Can you work these out from the model? Positions are in its coordinate system, mm. A direction names the side the tool comes from. Round coordinates to 2 decimals unless told otherwise and drop trailing zeros. Loops run counter-clockwise (first coordinate to the right, second up) from the corner with the lowest first, then second, coordinate; pieces in that order, holes last.
Autodesk Inventor part; units mm, degrees
ref_plane "YZ Plane" through (0, 0, 0) normal (1, 0, 0) x (0, 1, 0)
ref_plane "XZ Plane" through (0, 0, 0) normal (0, 1, 0) x (-1, 0, 0)
ref_plane "XY Plane" through (0, 0, 0) normal (0, 0, 1) x (1, 0, 0)
sketch "스케치1" plane through (0, 0, 0) normal (0, 1, 0) x (-1, 0, 0)
  line L0 (0, 0) -> (-59.6, 0)
  line L1 (-59.6, 0) -> (-59.6, 54.8)
  line L2 (-59.6, 54.8) -> (0, 54.8)
  line L3 (0, 54.8) -> (0, 0)
  dimension "d0" = 59.6
  dimension "d1" = 54.8
extrude "돌출1" add sketch "스케치1" along normal blind 14.7
sketch "스케치3" plane through (0, 14.7, 0) normal (0, 1, 0) x (1, 0, 0)
  line L0 (3.6, -3.85) -> (56, -3.85)
  line L1 (56, -3.85) -> (56, -50.95)
  line L2 (56, -50.95) -> (3.6, -50.95)
  line L3 (3.6, -50.95) -> (3.6, -3.85)
  point P0 (0, 0)
  dimension "d10" = 52.4
  dimension "d11" = 47.1
extrude "돌출2" add sketch "스케치3" along normal blind 7.2
sketch "스케치4" plane through (0, 21.9, 0) normal (0, 1, 0) x (1, 0, 0)
  line L0 (23.4801, -25.2454) -> (33.4417, -25.2454) construction
  line L1 (33.4417, -25.2454) -> (33.4417, -28.4935) construction
  line L2 (33.4417, -28.4935) -> (23.4801, -28.4935) construction
  line L3 (23.4801, -28.4935) -> (23.4801, -25.2454) construction
  line L4 (25.5376, -28.4293) -> (25.1523, -28.4293)
  line L5 (25.1523, -28.4293) -> (25.1523, -28.1773)
  spline S0 degree 2 poles (25.1523, -28.1773) (24.9745, -28.3329) (24.6558, -28.4935) (24.4582, -28.4935) knots 0 0 0 1 2 2 2
  spline S1 degree 2 poles (24.4582, -28.4935) (24.31, -28.4935) (24.0457, -28.3947) (23.9494, -28.2885) knots 0 0 0 1 2 2 2
  spline S2 degree 2 poles (23.9494, -28.2885) (23.8506, -28.1823) (23.7419, -27.8587) (23.7419, -27.6265) knots 0 0 0 1 2 2 2
  line L6 (23.7419, -27.6265) -> (23.7419, -26.142)
  line L7 (23.7419, -26.142) -> (24.1272, -26.142)
  line L8 (24.1272, -26.142) -> (24.1272, -27.4462)
  spline S3 degree 2 poles (24.1272, -27.4462) (24.1272, -27.629) (24.1544, -27.8686) (24.2013, -27.9575) knots 0 0 0 1 2 2 2
  spline S4 degree 2 poles (24.2013, -27.9575) (24.2483, -28.0464) (24.4088, -28.1279) (24.5595, -28.1279) knots 0 0 0 1 2 2 2
  spline S5 degree 2 poles (24.5595, -28.1279) (24.7003, -28.1279) (25.0189, -27.9674) (25.1523, -27.8513) knots 0 0 0 1 2 2 2
  line L9 (25.1523, -27.8513) -> (25.1523, -26.142)
  line L10 (25.1523, -26.142) -> (25.5376, -26.142)
  line L11 (25.5376, -26.142) -> (25.5376, -28.4293)
  spline S6 degree 2 poles (28.0126, -27.2486) (28.0126, -27.8093) (27.4692, -28.4935) (27.0591, -28.4935) knots 0 0 0 1 2 2 2
  spline S7 degree 2 poles (27.0591, -28.4935) (26.8739, -28.4935) (26.6096, -28.4021) (26.4812, -28.3231) knots 0 0 0 1 2 2 2
  line L12 (26.4812, -28.3231) -> (26.4565, -28.4293)
  line L13 (26.4565, -28.4293) -> (26.0958, -28.4293)
  line L14 (26.0958, -28.4293) -> (26.0958, -25.2454)
  line L15 (26.0958, -25.2454) -> (26.4812, -25.2454)
  line L16 (26.4812, -25.2454) -> (26.4812, -26.3816)
  spline S8 degree 2 poles (26.4812, -26.3816) (26.6269, -26.2507) (26.9653, -26.0778) (27.1802, -26.0778) knots 0 0 0 1 2 2 2
  spline S9 degree 2 poles (27.1802, -26.0778) (27.568, -26.0778) (28.0126, -26.6978) (28.0126, -27.2486) knots 0 0 0 1 2 2 2
  spline S10 degree 2 poles (27.6149, -27.2782) (27.6149, -26.8682) (27.3654, -26.4434) (27.0888, -26.4434) knots 0 0 0 1 2 2 2
  spline S11 degree 2 poles (27.0888, -26.4434) (26.9332, -26.4434) (26.6121, -26.5916) (26.4812, -26.7052) knots 0 0 0 1 2 2 2
  line L17 (26.4812, -26.7052) -> (26.4812, -28.0168)
  spline S12 degree 2 poles (26.4812, -28.0168) (26.6269, -28.0884) (26.8517, -28.1477) (26.985, -28.1477) knots 0 0 0 1 2 2 2
  spline S13 degree 2 poles (26.985, -28.1477) (27.279, -28.1477) (27.6149, -27.7302) (27.6149, -27.2782) knots 0 0 0 1 2 2 2
  line L18 (28.8054, -28.4293) -> (28.4201, -28.4293)
  line L19 (28.4201, -28.4293) -> (28.4201, -25.2454)
  line L20 (28.4201, -25.2454) -> (28.8054, -25.2454)
  line L21 (28.8054, -25.2454) -> (28.8054, -28.4293)
  spline S14 degree 2 poles (31.2508, -27.2856) (31.2508, -27.8636) (30.695, -28.4935) (30.2306, -28.4935) knots 0 0 0 1 2 2 2
  spline S15 degree 2 poles (30.2306, -28.4935) (29.7539, -28.4935) (29.2081, -27.8439) (29.2081, -27.2856) knots 0 0 0 1 2 2 2
  spline S16 degree 2 poles (29.2081, -27.2856) (29.2081, -26.7126) (29.7712, -26.0778) (30.2306, -26.0778) knots 0 0 0 1 2 2 2
  spline S17 degree 2 poles (30.2306, -26.0778) (30.695, -26.0778) (31.2508, -26.7101) (31.2508, -27.2856) knots 0 0 0 1 2 2 2
  spline S18 degree 2 poles (30.8531, -27.2856) (30.8531, -26.841) (30.5295, -26.4088) (30.2306, -26.4088) knots 0 0 0 1 2 2 2
  spline S19 degree 2 poles (30.2306, -26.4088) (29.9318, -26.4088) (29.6057, -26.841) (29.6057, -27.2856) knots 0 0 0 1 2 2 2
  spline S20 degree 2 poles (29.6057, -27.2856) (29.6057, -27.7179) (29.9318, -28.1625) (30.2306, -28.1625) knots 0 0 0 1 2 2 2
  spline S21 degree 2 poles (30.2306, -28.1625) (30.5271, -28.1625) (30.8531, -27.7253) (30.8531, -27.2856) knots 0 0 0 1 2 2 2
  line L22 (33.4219, -28.4293) -> (32.9501, -28.4293)
  line L23 (32.9501, -28.4293) -> (32.3944, -27.5697)
  line L24 (32.3944, -27.5697) -> (31.8238, -28.4293)
  line L25 (31.8238, -28.4293) -> (31.3866, -28.4293)
  line L26 (31.3866, -28.4293) -> (32.1795, -27.2955)
  line L27 (32.1795, -27.2955) -> (31.394, -26.142)
  line L28 (31.394, -26.142) -> (31.8658, -26.142)
  line L29 (31.8658, -26.142) -> (32.4191, -26.9942)
  line L30 (32.4191, -26.9942) -> (32.9847, -26.142)
  line L31 (32.9847, -26.142) -> (33.4219, -26.142)
  line L32 (33.4219, -26.142) -> (32.634, -27.2708)
  line L33 (32.634, -27.2708) -> (33.4219, -28.4293)
  point P0 (0, 0)
extrude "돌출3" cut sketch "스케치4" against normal blind 1.55
sketch "스케치5" plane through (0, 0, 54.8) normal (0, 0, 1) x (1, 0, 0)
  line L0 (14.8, 0) -> (44.8, 0)
  line L1 (44.8, 0) -> (44.8, 6)
  line L2 (44.8, 6) -> (14.8, 6)
  line L3 (14.8, 6) -> (14.8, 0)
  point P0 (0, 0)
  dimension "d16" = 30
  dimension "d17" = 6
sketch "스케치6" plane through (59.6, 0, 0) normal (0, 0, -1) x (-1, 0, 0)
  line L0 (44.8, 0) -> (14.8, 0)
  line L1 (14.8, 0) -> (14.8, 6)
  line L2 (14.8, 6) -> (44.8, 6)
  line L3 (44.8, 6) -> (44.8, 0)
  point P0 (59.6, 0)
  dimension "d18" = 30
  dimension "d19" = 6
extrude "돌출4" add sketch "스케치6" along normal blind 14.6
extrude "돌출5" add sketch "스케치5" along normal blind 14.6
sketch "스케치10" plane through (14.8, 6, 54.8) normal (0, 1, 0) x (1, 0, 0)
  circle A0 centre (15, -9.6) radius 2
  point P0 (-14.8, 54.8)
  dimension "d25" = 4
sketch "스케치12" plane through (14.8, 6, 0) normal (0, 1, 0) x (1, 0, 0)
  circle A0 centre (15, 9.6) radius 2
  point P0 (-14.8, 0)
  dimension "d27" = 4
extrude "돌출6" cut sketch "스케치10" against normal blind 70.15
extrude "돌출7" cut sketch "스케치12" against normal blind 104.1
properties part number "gps_antenna"
(1) Suppose I cut it at B-B (y = 5). Write out the boundary of the cut face in (x, z), then the cut area to 3 significant figures.
(2) Which directions (+Z, -Z, +X, -X, +Y, -Y) give clear straight access to the entire face, cutting with the end or side of a thin tool? Please do faces 5 (the flat face through (14.8, 3, 62)), 6 (the flat face through (56, 18, 27)), 7 (the flat face through (14.8, 3, -7)), 8 (the flat face through (30, 6, 62)).
(3) Suppose I cut it at D-D (z = 46). Write out the boundary of the cut face in (x, y).
(4) We'd pull the mould along X, two halves only. Please class faces 1 (the flat face through (29, 18, 3.85)), 2 (the flat face through (0, 7, 28)), 3 (the flat face through (32.4, 20.35, 27.3)), 4 (the flat face through (24, 20.35, 28)): released by +X, released by -X, zero draft, split by the parting line, or undercut.
(5) Suppose I cut it at A-A (z = 64.4). Write out the boundary of the cut face in (x, y).
(6) Suppose I cut it at C-C (x = 37.5). Write out the boundary of the cut face in (y, z).
(7) If I drill on line 1 (Z direction, x = 29.8, y = 4.15); line 2 (X direction, y = 2.5, z = 64.4); line 3 (Z direction, x = 46, y = 8), over which ranges is the centre line in solid material (lowest first)?
(8) For pin 1 (5 mm diameter, centred on y = 3, z = 65, fed in from +X); pin 2 (4.5 mm diameter, centred on x = 17.5, y = 9, fed in from -Z); pin 3 (0.5 mm diameter, centred on y = 21, z = 27.5, fed in from +X), each with a flat end and sliding along its axis, tell me the tip position at first contact or that it passes through.
Check result:
1. outline: (0, 0) - (14.8, 0) - (14.8, -14.6) - (44.8, -14.6) - (44.8, 0) - (59.6, 0) - (59.6, 54.8) - (44.8, 54.8) - (44.8, 69.4) - (14.8, 69.4) - (14.8, 54.8) - (0, 54.8) - close; hole circle Ø4 at (29.8, -9.6); hole circle Ø4 at (29.8, 64.4)
1. area: 4,120 mm2
2. face 5: +Z, -X, +Y, -Y
2. face 6: +Z, -Z, +X, +Y
2. face 7: -Z, -X, +Y, -Y
2. face 8: +Z, +X, -X, +Y
3. outline: (0, 0) - (59.6, 0) - (59.6, 14.7) - (56, 14.7) - (56, 21.9) - (3.6, 21.9) - (3.6, 14.7) - (0, 14.7) - close
4. face 1: zero draft
4. face 2: released by -X
4. face 3: undercut
4. face 4: undercut
5. outline: (14.8, 0) - (27.8, 0) - (27.8, 6) - (14.8, 6) - close; (31.8, 0) - (44.8, 0) - (44.8, 6) - (31.8, 6) - close
6. outline: (0, -14.6) - (6, -14.6) - (6, 0) - (14.7, 0) - (14.7, 3.85) - (21.9, 3.85) - (21.9, 50.95) - (14.7, 50.95) - (14.7, 54.8) - (6, 54.8) - (6, 69.4) - (0, 69.4) - close
7. line 1: z = -14.6 to -11.6, -7.6 to 62.4, 66.4 to 69.4
7. line 2: x = 14.8 to 27.8, 31.8 to 44.8
7. line 3: z = 0 to 54.8
8. pin 1: stops at x = 44.8
8. pin 2: stops at z = 0
8. pin 3: stops at x = 56
